The listing builds one solid part. Answer for the finished solid, in the listing's coordinates (mm). A direction names the side the tool comes from. Round coordinates to 2 decimals unless told otherwise and drop trailing zeros. Order: outer loops, then holes, each group sorted by start corner. A loop starts at its lowest first (then second) coordinate and runs counter-clockwise, first axis right, second up. Notation, with made-up numbers: (1.25, 5.25) -> (7.25, 5.25) arc R9 ccw to (7.25, 20.25) -> close; hole circle Ø2 at (-38.5, 88.25). An arc over 180 degrees is marked (long way). Answer in a Markdown table with one row per item. Add a question column.
```python
from build123d import *

# Parameters (mm, degrees)
SKETCH1_R                       = 0.75
BOSS_EXTRUDE1_DEPTH             = 1.7
SKETCH1_4_R                     = 1
BOSS_EXTRUDE2_DEPTH             = 0.3
BOSS_EXTRUDE3_DEPTH             = 11.4
BOSS_EXTRUDE4_REACH             = 24.984
CUT_EXTRUDE1_DEPTH              = 15.8
BOSS_EXTRUDE5_DEPTH             = 2
BOSS_EXTRUDE6_DEPTH             = 2
CUT_EXTRUDE4_DEPTH              = 10
CUT_EXTRUDE4_DEPTH_BACK         = 12
BOSS_EXTRUDE7_REACH             = 31.456
BOSS_EXTRUDE7_DIRECTION_2_REACH = 31.456
FILLET1_R                       = 0.5


with BuildPart() as part:
    # Sketch1 → Boss-Extrude1 (new body)
    with BuildSketch(Plane(origin=(0, 0, 0), x_dir=(1, 0, 0), z_dir=(0, 1, 0))):
        Polygon((13.4, 2.5), (-4.4, 2.5), (-4.4, 0), (-6.4, 0), (-6.4, -1.5), (15.4, -1.5), (15.4, 0), (13.4, 0), align=None)
        with Locations(Location((3, 0, 0), (0, 0, 270))):
            Circle(SKETCH1_R, mode=Mode.SUBTRACT)
        with Locations(Location((6, 0, 0), (0, 0, 270))):
            Circle(SKETCH1_R, mode=Mode.SUBTRACT)
        with Locations(Location((9, 0, 0), (0, 0, 270))):
            Circle(SKETCH1_R, mode=Mode.SUBTRACT)
        with Locations(Location((0, 0, 0), (0, 0, 270))):
            Circle(SKETCH1_R, mode=Mode.SUBTRACT)
    extrude(amount=BOSS_EXTRUDE1_DEPTH)

    # Sketch1<4> → Boss-Extrude2 (add)
    with BuildSketch(Plane(origin=(0, 0, 0), x_dir=(1, 0, 0), z_dir=(0, 1, 0))):
        Polygon((13.4, 2.5), (-4.4, 2.5), (-4.4, 0), (-6.4, 0), (-6.4, -1.5), (15.4, -1.5), (15.4, 0), (13.4, 0), align=None)
        with Locations(Location((0, 0, 0), (0, 0, 270))):
            Circle(SKETCH1_4_R, mode=Mode.SUBTRACT)
        with Locations(Location((3, 0, 0), (0, 0, 270))):
            Circle(SKETCH1_4_R, mode=Mode.SUBTRACT)
        with Locations(Location((6, 0, 0), (0, 0, 270))):
            Circle(SKETCH1_4_R, mode=Mode.SUBTRACT)
        with Locations(Location((9, 0, 0), (0, 0, 270))):
            Circle(SKETCH1_4_R, mode=Mode.SUBTRACT)
    extrude(amount=-BOSS_EXTRUDE2_DEPTH)

    # Sketch1<7> → Boss-Extrude3 (add)
    with BuildSketch(Plane(origin=(0, 0, 0), x_dir=(1, 0, 0), z_dir=(0, 1, 0))):
        Polygon((13.4, 1), (13.4, 2.5), (-4.4, 2.5), (-4.4, 1), (-2.4, 1), (0, 1), (3, 1), (6, 1), (9.000000004, 1), (11.4, 1), align=None)
        Polygon((-2.4, 1), (-4.4, 1), (-4.4, 0), (-6.4, 0), (-6.4, -1.5), (-2.4, -1.5), align=None)
        Polygon((13.4, 0), (13.4, 1), (11.4, 1), (11.4, -1.5), (15.4, -1.5), (15.4, 0), align=None)
    extrude(amount=BOSS_EXTRUDE3_DEPTH)

    # Boss-Extrude4: up to this face of the body (flat: up to its plane)
    boss_extrude4_end = Plane(part.part.faces().sort_by_distance((15.4, 5.55, 0.75))[0])
    # Sketch2 → Boss-Extrude4 (add, up to the picked face)
    with BuildSketch(Plane.ZY.offset(4.4), mode=Mode.PRIVATE) as boss_extrude4_sk1:
        Polygon((0.5, 21.4), (-2.5, 11.4), (1.5, 11.4), (4.2, 20.4), (1.7, 20.4), (2, 21.4), align=None)
    boss_extrude4_tool1 = split(extrude(boss_extrude4_sk1.sketch, amount=-BOSS_EXTRUDE4_REACH, mode=Mode.PRIVATE), bisect_by=boss_extrude4_end, keep=Keep.BOTH, mode=Mode.PRIVATE)
    add(boss_extrude4_tool1.solids().sort_by(Axis((-4.4, 16.1, 0.86), (1, 0, 0)))[0])

    # Sketch2<5> → Cut-Extrude1 (cut)
    with BuildSketch(Plane.ZY.offset(4.4)):
        Polygon((1.7, 20.4), (-1, 11.4), (1.5, 11.4), (4.2, 20.4), align=None)
    extrude(amount=-CUT_EXTRUDE1_DEPTH, mode=Mode.SUBTRACT)

    # Sketch2<6> → Boss-Extrude5 (add)
    with BuildSketch(Plane.ZY.offset(4.4)):
        Polygon((1.7, 20.4), (-1, 11.4), (1.5, 11.4), (4.2, 20.4), align=None)
    extrude(amount=-BOSS_EXTRUDE5_DEPTH)

    # Sketch2<7> → Boss-Extrude6 (add)
    with BuildSketch(Plane.ZY.offset(4.4)):
        Polygon((0.5, 21.4), (-2.5, 11.4), (1.5, 11.4), (4.2, 20.4), (1.7, 20.4), (2, 21.4), align=None)
    extrude(amount=BOSS_EXTRUDE6_DEPTH)

    # Sketch5 → Cut-Extrude4 (cut, two sides: drawn at the far end of the back side and taken through both)
    with BuildSketch(Plane(origin=(0, 19.770642202, 5.931192661), x_dir=(1, 0, 0), z_dir=(0, 0.9578262852211515, 0.2873478855663452)).offset(-CUT_EXTRUDE4_DEPTH_BACK)):
        with BuildLine():
            ThreePointArc((-6.6, 4.689132716), (-5.561967393, 5.205345242), (-4.5, 5.670331609))
            Line((-4.5, 5.670331609), (-17.5, 5.670331609))
            Line((-17.5, 5.670331609), (-17.5, -7.329668391))
            ThreePointArc((-17.5, -7.329668391), (-17.035013633, -6.267700999), (-16.518801108, -5.229668391))
            ThreePointArc((-16.518801108, -5.229668391), (-12.307736314, 0.478067922), (-6.6, 4.689132716))
        make_face()
        with BuildLine():
            ThreePointArc((25.518801108, -5.229668391), (26.035013633, -6.267700999), (26.5, -7.329668391))
            Line((26.5, -7.329668391), (26.5, 5.670331609))
            Line((26.5, 5.670331609), (13.5, 5.670331609))
            ThreePointArc((13.5, 5.670331609), (14.561967393, 5.205345242), (15.6, 4.689132716))
            ThreePointArc((15.6, 4.689132716), (21.307736314, 0.478067922), (25.518801108, -5.229668391))
        make_face()
    extrude(amount=CUT_EXTRUDE4_DEPTH + CUT_EXTRUDE4_DEPTH_BACK, mode=Mode.SUBTRACT)

    # Boss-Extrude7: up to this face of the body (flat: up to its plane)
    boss_extrude7_end = Plane(part.part.faces().sort_by_distance((-6.4, 12.005993792, 1.097626434))[0])
    # Sketch2<8> → Boss-Extrude7 (add, up to the picked face)
    with BuildSketch(Plane.ZY.offset(4.4), mode=Mode.PRIVATE) as boss_extrude7_sk1:
        Polygon((4.5, 21.4), (2, 21.4), (1.7, 20.4), (4.2, 20.4), align=None)
    boss_extrude7_tool1 = split(extrude(boss_extrude7_sk1.sketch, amount=BOSS_EXTRUDE7_REACH, mode=Mode.PRIVATE), bisect_by=boss_extrude7_end, keep=Keep.BOTH, mode=Mode.PRIVATE)
    add(boss_extrude7_tool1.solids().sort_by(Axis((-4.4, 20.9, 3.1), (-1, 0, 0)))[0])

    # Boss-Extrude7 direction 2: up to this face of the body (flat: up to its plane)
    boss_extrude7_direction_2_end = Plane(part.part.faces().sort_by_distance((15.4, 12.005993792, 1.097626434))[0])
    # Sketch2<8> → Boss-Extrude7 direction 2 (add, up to the picked face)
    with BuildSketch(Plane.ZY.offset(4.4), mode=Mode.PRIVATE) as boss_extrude7_direction_2_sk1:
        Polygon((4.5, 21.4), (2, 21.4), (1.7, 20.4), (4.2, 20.4), align=None)
    boss_extrude7_direction_2_tool1 = split(extrude(boss_extrude7_direction_2_sk1.sketch, amount=-BOSS_EXTRUDE7_DIRECTION_2_REACH, mode=Mode.PRIVATE), bisect_by=boss_extrude7_direction_2_end, keep=Keep.BOTH, mode=Mode.PRIVATE)
    add(boss_extrude7_direction_2_tool1.solids().sort_by(Axis((-4.4, 20.9, 3.1), (1, 0, 0)))[0])

    # Fillet1
    fillet1_edges = [part.edges().sort_by_distance(p)[0] for p in [
        (4.5, 21.4, 0.5),
        (14.46035786, 21.4, 0.936198075),
        (-5.46035786, 21.4, 0.936198075),
    ]]
    fillet(fillet1_edges, radius=FILLET1_R)


solid = part.part
```
1. For faces 4 (the flat face through (11.4, 11, 1)), 5 (the cylindrical face through (2.335, 0.838, 0.346)), 6 (the flat face through (4, 21.4, 3)), determine the directions among +Z, -Z, +X, -X, +Y, -Y from which every point of the face is accessible in a straight line to the end or side of a thin tool.
2. Straight lines are drawn through the part: line 1 along X through (y, z) = (15, 1); line 2 along Z through (x, y) = (10, 10); line 3 along X through (y, z) = (10, -1.5). For each, find the intervals that lie inside material, in ascending order.
3. The part is cut by section A-A (x = 9). Give the vertices of the cut face in (y, z).
4. Each of these flat-tipped pins is pushed along its axis until it touches: pin 1 (0.8 mm diameter, centred on y = 7, z = -1, fed in from +X); pin 2 (2 mm diameter, centred on x = 14.5, y = 5.5, fed in from -Z); pin 3 (1.2 mm diameter, centred on x = 0, z = 0, fed in from +Y). Where does it stop, or does it pass through?
5. The part is cut by section D-D (z = 3.5). Give the vertices of the cut face in (x, y), then the cut area to 3 significant figures.
6. The mould has two halves that part along Z. Classify faces 1 (the cylindrical face through (9.632, 0.838, 0.403)), 2 (the flat face through (14, 11.4, -1)), 3 (the flat face through (14, 5, 0)): released by +Z, released by -Z, zero draft, split by the parting line, or undercut.
7. The part is cut by section C-C (y = 10). Give the vertices of the cut face in (x, z).
8. The part is cut by section B-B (z = 2.25). Give the vertices of the cut face in (x, y), then the cut area to 3 significant figures.
Report:
| question | item | result |
|---|---|---|
| 1 | face 4 | +Z |
| 1 | face 5 | -Y |
| 1 | face 6 | +Z, -Z, +X, -X, +Y |
| 2 | line 1 | x = -6.4 to -2.4, 11.4 to 15.4 |
| 2 | line 2 | z = -2.5 to -1 |
| 2 | line 3 | x = -4.4 to 13.4 |
| 3 | outline | (-0.3, -2.5) -> (11.4, -2.5) -> (21.04, 0.39) arc R0.5 ccw to (21.4, 0.87) -> (21.4, 4.5) -> (20.4, 4.2) -> (20.4, 1.7) -> (11.4, -1) -> (1.7, -1) -> (1.7, -0.75) -> (0, -0.75) -> (0, -1) -> (-0.3, -1) -> close; (-0.3, 1) -> (0, 1) -> (0, 0.75) -> (1.7, 0.75) -> (1.7, 1.5) -> (-0.3, 1.5) -> close |
| 4 | pin 1 | stops at x = 13.4 |
| 4 | pin 2 | stops at z = 0 |
| 4 | pin 3 | stops at y = 21.32 |
| 5 | outline | (-6.4, 18.07) -> (-2.4, 18.07) -> (-2.4, 20.4) -> (11.4, 20.4) -> (11.4, 18.07) -> (15.4, 18.07) -> (15.4, 21.4) -> (-6.4, 21.4) -> close |
| 5 | area | 40.5 mm^2 |
| 6 | face 1 | undercut |
| 6 | face 2 | zero draft |
| 6 | face 3 | released by -Z |
| 7 | outline | (-6.4, 0) -> (-4.4, 0) -> (-4.4, -2.5) -> (13.4, -2.5) -> (13.4, 0) -> (15.4, 0) -> (15.4, 1.5) -> (11.4, 1.5) -> (11.4, -1) -> (-2.4, -1) -> (-2.4, 1.5) -> (-6.4, 1.5) -> close |
| 8 | outline | (-6.4, 13.9) -> (-2.4, 13.9) -> (-2.4, 20.4) -> (11.4, 20.4) -> (11.4, 13.9) -> (15.4, 13.9) -> (15.4, 21.4) -> (-6.4, 21.4) -> close |
| 8 | area | 73.8 mm^2 |
